from build123d import *

# Parameters (mm, degrees)
BOSS_EXTRUDE1_DEPTH       = 50
CUT_EXTRUDE1_DEPTH        = 30
F_3_0MM_DOWEL_HOLE1_D     = 3
F_3_0MM_DOWEL_HOLE1_DEPTH = 6
F_3_0MM_DOWEL_HOLE1_TIP   = 0.901290929
M5_CLEARANCE_HOLE1_D      = 5.5


with BuildPart() as part:
    # Sketch1 → Revolve1 (revolve)
    with BuildSketch(Plane.XY, mode=Mode.PRIVATE) as revolve1_sk:
        Polygon((-24, 0), (-24, 50), (-16, 50), (-16, 34), (-13, 34), (-13, 30), (-16, 30), (-20, 30), (-20, 0), align=None)
    revolve(revolve1_sk.sketch.rotate(Axis((0, 0, 0), (0, 1, 0)), 270), axis=Axis((0, 0, 0), (0, 1, 0)))

    # Sketch6 → Boss-Extrude1 (add)
    with BuildSketch(Plane(origin=(0, 50, 0), x_dir=(1, 0, 0), z_dir=(0, 1, 0))):
        with BuildLine():
            Line((0, -24), (20.5, -24))
            ThreePointArc((20.5, -24), (27.571067812, -21.071067812), (30.5, -14))
            Line((30.5, -14), (30.5, 14))
            ThreePointArc((30.5, 14), (27.571067812, 21.071067812), (20.5, 24))
            Line((20.5, 24), (0, 24))
            ThreePointArc((0, 24), (24, 0), (0, -24))
        make_face()
    extrude(amount=-BOSS_EXTRUDE1_DEPTH)

    # Sketch5 → Cut-Extrude1 (cut)
    with BuildSketch(Plane(origin=(0, 0, 0), x_dir=(1, 0, 0), z_dir=(0, 1, 0))):
        Polygon((15.085272612, -18.666401641), (20.483393436, -35.301209276), (-37.381072525, -18.770693037), (-37.381072525, 22.982117566), (-6.915364934, 22.982117566), (0, 0), align=None)
    extrude(amount=CUT_EXTRUDE1_DEPTH, mode=Mode.SUBTRACT)

    # Ø3.0mm Dowel Hole1
    with Locations(Plane(origin=(0, 0, 0), x_dir=(-1, 0, 0), z_dir=(0, -1, 0))):
        with Locations((-24.5, -9), (-24.5, 9)):
            Hole(F_3_0MM_DOWEL_HOLE1_D / 2, depth=F_3_0MM_DOWEL_HOLE1_DEPTH)
            with Locations((0, 0, -(F_3_0MM_DOWEL_HOLE1_DEPTH + F_3_0MM_DOWEL_HOLE1_TIP / 2))):  # 118° drill point
                Cone(0, F_3_0MM_DOWEL_HOLE1_D / 2, F_3_0MM_DOWEL_HOLE1_TIP, mode=Mode.SUBTRACT)

    # M5 Clearance Hole1 (through all)
    with Locations(Plane(origin=(0, 0, 0), x_dir=(-1, 0, 0), z_dir=(0, -1, 0))):
        with Locations((-22.5, -16), (-22.5, 16)):
            Hole(M5_CLEARANCE_HOLE1_D / 2)


solid = part.part
For this review, take the finished solid that the model builds, in its own axes (mm). A direction names the side the tool comes from. Coordinates: 2 decimals unless noted, no trailing zeros. Order: outer loops, then holes, each group sorted by start corner. A loop starts at its lowest first (then second) coordinate and runs counter-clockwise, first axis right, second up. Notation, with made-up numbers: (52.25, 36) -> (68.25, 36) arc R24 cw to (68.25, 50) -> close; hole circle Ø5 at (54.25, -10.75). An arc over 180 degrees is marked (long way). Return JSON: item names as keys, results as strings.
1. We need section A-A on y = 5. Write out the cut boundary in (x, z), and give its area (3 significant figures).
Answer block:
{"outline": "(-6.92, -22.98) arc R24 ccw to (0, -24) -> (20.5, -24) arc R10 ccw to (30.5, -14) -> (30.5, 14) arc R10 ccw to (20.5, 24) -> (16.82, 24) -> (15.09, 18.67) -> (12.57, 15.56) arc R20 cw to (-5.76, -19.15) -> close; hole circle Ø5.5 at (22.5, -16); hole circle Ø5.5 at (22.5, 16); hole circle Ø3 at (24.5, -9); hole circle Ø3 at (24.5, 9)", "area": "667 mm²"}
2. We need section B-B on z = 0. Write out the cut boundary in (x, y), and give its area (3 significant figures).
Answer block:
{"outline": "(-24, 30) -> (-13, 30) -> (-13, 34) -> (-16, 34) -> (-16, 50) -> (-24, 50) -> close; (13, 30) -> (20, 30) -> (20, 0) -> (30.5, 0) -> (30.5, 50) -> (16, 50) -> (16, 34) -> (13, 34) -> close", "area": "789 mm²"}
3. We need section C-C on y = 26. Write out the cut boundary in (x, z).
Answer block:
{"outline": "(-6.92, -22.98) arc R24 ccw to (0, -24) -> (20.5, -24) arc R10 ccw to (30.5, -14) -> (30.5, 14) arc R10 ccw to (20.5, 24) -> (16.82, 24) -> (15.09, 18.67) -> (12.57, 15.56) arc R20 cw to (-5.76, -19.15) -> close; hole circle Ø5.5 at (22.5, -16); hole circle Ø5.5 at (22.5, 16)"}
4. Machinability: for faces 5 (the cylindrical face through (23, 3, -9)), 6 (the cylindrical face through (15.62, 41.89, 3.47)), 7 (the cylindrical face through (19.753, 25.35, 15.879)), 8 (the flat face through (15.94, 14.79, 21.3)), which of the approach directions +Z, -Z, +X, -X, +Y, -Y give a long, thin tool a straight path to every point of the face, cutting with its end or side? Answer none if there is none.
Answer block:
{"face 5": "-Y", "face 6": "+Y", "face 7": "+Y, -Y", "face 8": "+Z, -X, -Y"}
5. For line 1 (X direction, y = 31.8, z = 0); line 2 (X direction, y = 45, z = 0); line 3 (Y direction, x = 10, z = -9), list the stretches that pass through material, from the lowest coordinate up. Write a range as from..to.
Answer block:
{"line 1": "-24..-13, 13..30.5", "line 2": "-24..-16, 16..30.5", "line 3": "30..34"}
6. We need section D-D on y = 42.5. Write out the cut boundary in (x, z).
Answer block:
{"outline": "(0, -24) -> (20.5, -24) arc R10 ccw to (30.5, -14) -> (30.5, 14) arc R10 ccw to (20.5, 24) -> (0, 24) arc R24 ccw to start; hole circle Ø32 at (0, 0); hole circle Ø5.5 at (22.5, -16); hole circle Ø5.5 at (22.5, 16)"}
7. For pin 1 Ø4 at (x, y) = (24, 13) entering from -Z; pin 2 Ø3 at (x, z) = (-4, 13.5) entering from +Y; pin 3 Ø12 at (x, y) = (-18, 35) entering from +Z; pin 4 Ø7 at (x, z) = (22.5, -16) entering from -Y, all flat-tipped, find the tip position at first contact; note any pin that passes through.
Answer block:
{"pin 1": "z = -23.89", "pin 2": "y = 34", "pin 3": "z = 20.78", "pin 4": "y = 0"}
8. The part is to be moulded in two halves that separate along X. For faces 1 (the flat face through (10, 25, -24)), 2 (the flat face through (-6.347, 14.79, -21.094)), 3 (the cylindrical face through (27.49, 25.35, 21.15)), 4 (the cylindrical face through (23, 3, 9)), say which applies: +X half, -X half, draft (parallel to the pull), parting line (faces both ways), or undercut.
Answer block:
{"face 1": "draft", "face 2": "-X half", "face 3": "+X half", "face 4": "undercut"}
